The model under review builds one solid part; all positions refer to its coordinate system, in mm. Face numbers are marked on the shaded views. A direction names the side the tool comes from. Give positions to 0.01 mm unless a question says otherwise; leave off trailing zeros. Write each loop counter-clockwise with the first axis right and the second up, starting at its lowest first coordinate (ties: lowest second). Pieces come first, ordered by that corner, then holes. Notation, with made-up numbers: M 25,71.25 L 76,71.25 A23 ccw 76,80.25 Z; hole C 9,56.5 d10. An arc over 180 degrees is marked long. Write item = value, one per line. Start each with the question number.
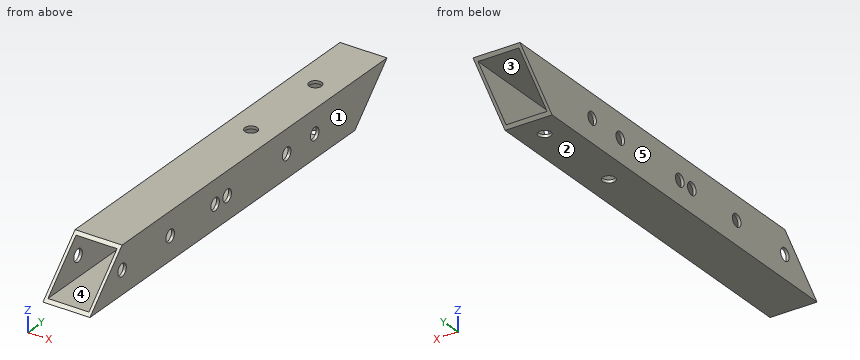
Autodesk Inventor part; units mm, degrees
ref_plane "YZ Plane" through (0, 0, 0) normal (1, 0, 0) x (0, 1, 0)
ref_plane "XZ Plane" through (0, 0, 0) normal (0, 1, 0) x (-1, 0, 0)
ref_plane "XY Plane" through (0, 0, 0) normal (0, 0, 1) x (1, 0, 0)
sketch "Sketch1" plane through (0, 0, 0) normal (0, 1, 0) x (-1, 0, 0)
  line L0 (0, 0) -> (25.4, 0)
  line L1 (25.4, 0) -> (25.4, 25.4)
  line L2 (25.4, 25.4) -> (0, 25.4)
  line L3 (0, 25.4) -> (0, 0)
  line L4 (1.5875, 23.8125) -> (23.8125, 23.8125)
  line L5 (23.8125, 23.8125) -> (23.8125, 1.5875)
  line L6 (23.8125, 1.5875) -> (1.5875, 1.5875)
  line L7 (1.5875, 1.5875) -> (1.5875, 23.8125)
  dimension "d0" = 25.4
  dimension "d2" = 25.4
  dimension "d3" = 1.5875
extrude "Extrusion1" add sketch "Sketch1" along normal blind 254
sketch "Sketch2" plane through (-25.4, 0, 0) normal (-1, 0, 0) x (0, 0, 1)
  line L0 (0, 254) -> (25.4, 254)
  line L1 (0, 0) -> (0, 254)
  line L2 (25.4, 0) -> (25.4, 254)
  line L3 (25.4, 234.95) -> (0, 209.55)
  point P0 (0, 228.6)
  dimension "d6" = 25.4
  dimension "d13" = 25.4
  dimension "d14" = 19.05
extrude "Extrusion2" cut sketch "Sketch2" against normal blind 25.4
sketch "Sketch3" plane through (-25.4, 0, 0) normal (-1, 0, 0) x (0, 0, 1)
  line L0 (25.4, 254) -> (0, 228.6)
  line L1 (0, 0) -> (25.4, 0)
  line L2 (25.4, 0) -> (25.4, 234.95)
  line L3 (0, 0) -> (25.4, 25.4)
extrude "Extrusion3" cut sketch "Sketch3" against normal blind 25.4
sketch "Sketch4" plane through (-25.4, 25.4, 25.4) normal (-1, 0, 0) x (0, 0, 1)
  circle A0 centre (-12.7, 38.1) radius 3.3782
  circle A1 centre (-12.7, 0) radius 3.3782
extrude "Extrusion4" cut sketch "Sketch4" against normal blind 25.4
sketch "Sketch5" plane through (0, 209.55, 0) normal (0, 0, -1) x (-1, 0, 0)
  circle A0 centre (12.7, -12.7) radius 3.3782
  circle A1 centre (12.7, -63.5) radius 3.3782
extrude "Extrusion5" cut sketch "Sketch5" against normal blind 25.4
sketch "Sketch6" plane through (0, 0, 0) normal (1, 0, 0) x (0, 0, -1)
  circle A0 centre (-12.7, 177.8) radius 3.3782
  circle A1 centre (-12.7, 155.575) radius 3.3782
extrude "Extrusion6" cut sketch "Sketch6" against normal blind 25.4
sketch "Sketch7" plane through (-25.4, 25.4, 25.4) normal (-1, 0, 0) x (0, 0, 1)
  circle A0 centre (-12.7, 83.1396) radius 3.3782
  circle A1 centre (-12.7, 73.6146) radius 3.3782
extrude "Extrusion7" cut sketch "Sketch7" against normal blind 25.4
properties part number "Square Tube 3" material "Aluminum 6061"
Item 1: For the marked faces 4 and 5, list the 3-axis set-ups (+Z, -Z, +X, -X, +Y, -Y) from which the entire face can be reached by the end or side of a thin tool; tool diameter is ignored.
Item 2: Clearance check with a flat-ended pin moving along its axis: P1, Ø5.5, axis at y = 63.5, z = 12.7, coming from the +X side. State where the tip first meets the part, or that it passes through.
Item 3: We need section D-D, the plane z = 12.7. Give the number of separate pieces and of enclosed holes in the cut face, and give its area (3 significant figures).
Item 4: We need section A-A, the plane x = -12.7. Write out the cut boundary in (y, z).
Item 5: We need section C-C, the plane y = 32. Write out the cut boundary in (x, z), and give its area (3 significant figures).
Item 6: To check wall thickness, follow probe 1 along X at (y, z) = (138, 20); probe 2 along Z at (x, y) = (-11.25, 38.5); probe 3 along Y at (x, z) = (-12.7, 24.35). State the ranges of each line that lie inside material, in increasing order. Write a range as [from, to].
Item 7: The part is to be moulded in two halves that separate along Z. For the marked faces 1, 2 and 3, say which applies: released by +Z, released by -Z, zero draft, split by the parting line, or undercut.
Item 8: We need section B-B, the plane y = 177.8. Write out the cut boundary in (x, z).
Worked out:
q1.face_4 = +Y, -Y
q1.face_5 = +Z, -Z, -X, +Y, -Y
q2.P1 = through
q3.separate_pieces = 14
q3.enclosed_holes = 0
q3.area = 537 mm²
q4.outline = M 0,0 L 142.67,0 L 142.67,1.59 L 1.59,1.59 Z; M 23.81,23.81 L 142.67,23.81 L 142.67,25.4 L 25.4,25.4 Z; M 149.43,0 L 193.47,0 L 193.47,1.59 L 149.43,1.59 Z; M 149.43,23.81 L 193.47,23.81 L 193.47,25.4 L 149.43,25.4 Z; M 200.23,0 L 209.55,0 L 211.14,1.59 L 200.23,1.59 Z; M 200.23,23.81 L 233.36,23.81 L 234.95,25.4 L 200.23,25.4 Z
q5.outline = M -25.4,0 L 0,0 L 0,25.4 L -25.4,25.4 Z; hole M -23.81,1.59 L -1.59,1.59 L -1.59,23.81 L -23.81,23.81 Z
q5.area = 151 mm²
q6.probe_1 = [-25.4, -23.81], [-1.59, 0]
q6.probe_2 = [0, 1.59], [23.81, 25.4]
q6.probe_3 = [24.35, 142.67], [149.43, 193.47], [200.23, 233.9]
q7.face_1 = zero draft
q7.face_2 = released by -Z
q7.face_3 = undercut
q8.outline = M -25.4,0 L 0,0 L 0,9.32 L -1.59,9.32 L -1.59,1.59 L -23.81,1.59 L -23.81,9.32 L -25.4,9.32 Z; M -25.4,16.08 L -23.81,16.08 L -23.81,23.81 L -1.59,23.81 L -1.59,16.08 L 0,16.08 L 0,25.4 L -25.4,25.4 Z
